```python
from build123d import *

# Parameters (mm, degrees)
F0_W        = 12.9503121972
F0_H        = 15
F0_R        = 1
F0_W_2      = 1.5692040324
F1_DEPTH    = 5
F2_DEPTH    = 2
F0_H_2      = 0.5759084597
F0_H_3      = 0.5869377777
F3_DEPTH    = 35
F4_T1_DEPTH = 34.3491316119


# Not quite as in the source:
# - a fillet or chamfer that OpenCascade refuses, or shapes differently, is made with other operations: its cross-section is extruded or revolved along the edge and cut away or added
# - a feature names something its author has since deleted; it is built from what else it names


with BuildPart() as f1:
    # F0 (on Front) → F1 (new body)
    with BuildSketch(Plane.XZ):
        with Locations((-28.5248439014, 7.5)):
            Rectangle(F0_W, F0_H)
        Polygon((20.4804837704, 0), (20.4804837704, 15), (-20.4804837704, 15), (-20.4804837704, 0), (-20, 0), (-20, -15), (20, -15), (20, 0), align=None)
        Circle(F0_R, mode=Mode.SUBTRACT)
        with Locations((-21.2650857866, 7.5)):
            Rectangle(F0_W_2, F0_H)
        with Locations((21.2650857866, 7.5)):
            Rectangle(F0_W_2, F0_H)
        with Locations((28.5248439014, 7.5)):
            Rectangle(F0_W, F0_H)
        Circle(F0_R)
    extrude(amount=F1_DEPTH)

    # F0 (on Front) → F2 (join)
    with BuildSketch(Plane.XZ):
        Circle(F0_R)
    extrude(amount=-F2_DEPTH)

    # F0 (on Front) → F3 (join)
    with BuildSketch(Plane.XZ):
        with Locations((-21.2650857866, 7.5)):
            Rectangle(F0_W_2, F0_H)
        with Locations((-21.2650857866, -0.2879542299)):
            Rectangle(F0_W_2, F0_H_2)
        with Locations((-21.2650857866, 15.2934688888)):
            Rectangle(F0_W_2, F0_H_3)
        with Locations((21.2650857866, 15.2934688888)):
            Rectangle(F0_W_2, F0_H_3)
        with Locations((21.2650857866, 7.5)):
            Rectangle(F0_W_2, F0_H)
        with Locations((21.2650857866, -0.2879542299)):
            Rectangle(F0_W_2, F0_H_2)
    extrude(amount=F3_DEPTH)

    # F4: fillet of radius 5 on 2 edges, made by hand

    # F4_s2 → F4_t1 (cut)
    with BuildSketch(Plane.XY.offset(-9.669051147)):
        with BuildLine():
            ThreePointArc((-22.0496878028, -31.3627429251), (-21.6406561014, -33.3434019268), (-20.4804837704, -35))
            Line((-20.4804837704, -35), (-22.0496878028, -35))
            Line((-22.0496878028, -35), (-22.0496878028, -31.3627429251))
        make_face()
        with BuildLine():
            ThreePointArc((20.4804837704, -35), (21.6406561014, -33.3434019268), (22.0496878028, -31.3627429251))
            Line((22.0496878028, -31.3627429251), (22.0496878028, -35))
            Line((22.0496878028, -35), (20.4804837704, -35))
        make_face()
    extrude(amount=F4_T1_DEPTH, mode=Mode.SUBTRACT)


solid = f1.part
```
The model under review builds one solid part; all positions refer to its coordinate system, in mm. A direction names the side the tool comes from. Round coordinates to 2 decimals unless told otherwise and drop trailing zeros. Write each loop counter-clockwise with the first axis right and the second up, starting at its lowest first coordinate (ties: lowest second). Pieces come first, ordered by that corner, then holes. Notation, with made-up numbers: (-30, -37) - (23, -37) arc R28 cw to (23, 0) - close; hole circle Ø10 at (-17, 16.25). An arc over 180 degrees is marked (long way). Answer as CSV lines item,"result". Start each with the question number.
(1) To check wall thickness, follow line 1 (X direction, y = -26, z = 6); line 2 (Y direction, x = 2.5, z = 14); line 3 (Z direction, x = -23, y = -2.5). State the ranges of each line that lie inside material, in increasing order.
(2) We need section C-C on x = 0. State the section outline as (y, z) points, plus the area to 3 significant figures.
(3) For faces 1 (the flat face through (29, -2, 15)), 2 (the flat face through (-29, -2, 0)), 3 (the flat face through (28, -5, 8)), list the 3-axis set-ups (+Z, -Z, +X, -X, +Y, -Y) from which the entire face can be reached by the end or side of a thin tool; tool diameter is ignored.
(4) We need section B-B on z = 4. State the section outline as (x, y) points.
(5) For pin 1 Ø4 at (y, z) = (-3.5, -5) entering from -X; pin 2 Ø1.3 at (x, y) = (21, -12) entering from -Z; pin 3 Ø5.5 at (x, y) = (-8.5, -2.5) entering from +Z; pin 4 Ø5 at (y, z) = (-8, -11) entering from +X (1 decimal), all flat-tipped, find the tip position at first contact; note any pin that passes through.
(6) We need section A-A on y = -20.5. State the section outline as (x, z) points.
(7) We need section D-D on x = 23. State the section outline as (y, z) points.
(8) Draft analysis for pull direction X (two halves, no side actions). For faces 4 (the flat face through (21, -17, 15.587)), 5 (the flat face through (0, -2, 15)), 6 (the flat face through (-35, -2, 7)), 7 (the flat face through (20.48, -21, 8)), state which applies: pulls with the +X half, pulls with the -X half, needs draft (parallel to the pull), parting line crosses it, or undercut.
Worked answers:
1,line 1,"-22.05 to -20.48, 20.48 to 22.05"
1,line 2,"-5 to 0"
1,line 3,"0 to 15"
2,outline,"(-5, -15) - (0, -15) - (0, -1) - (2, -1) - (2, 1) - (0, 1) - (0, 15) - (-5, 15) - close"
2,area,"154 mm²"
3,face 1,"+Z, +X, +Y, -Y"
3,face 2,"-Z, -X, +Y, -Y"
3,face 3,"+Z, -Z, +X, -Y"
4,outline,"(-35, -5) - (-22.05, -5) - (-22.05, -31.36) arc R5 ccw to (-20.48, -35) - (-20.48, -5) - (20.48, -5) - (20.48, -35) arc R5 ccw to (22.05, -31.36) - (22.05, -5) - (35, -5) - (35, 0) - (-35, 0) - close"
5,pin 1,"x = -20"
5,pin 2,"z = -0.58"
5,pin 3,"z = 15"
5,pin 4,"through"
6,outline,"(-22.05, -0.58) - (-20.48, -0.58) - (-20.48, 15.59) - (-22.05, 15.59) - close; (20.48, -0.58) - (22.05, -0.58) - (22.05, 15.59) - (20.48, 15.59) - close"
7,outline,"(-5, 0) - (0, 0) - (0, 15) - (-5, 15) - close"
8,face 4,"needs draft"
8,face 5,"undercut"
8,face 6,"pulls with the -X half"
8,face 7,"undercut"
